from build123d import *

# Parameters (mm, degrees)
SKETCH1_R           = 2.38125
BOSS_EXTRUDE1_DEPTH = 38.1
FILLET1_R           = 2.54
SKETCH2_R           = 6.35
CUT_EXTRUDE1_DEPTH  = 19.05


with BuildPart() as part:
    # Sketch1 → Boss-Extrude1 (new body)
    with BuildSketch(Plane(origin=(0, 0, 0), x_dir=(1, 0, 0), z_dir=(0, 1, 0))):
        with BuildLine():
            Line((216.9989119, 96.687544883), (-5.2510881, 14.137544883))
            ThreePointArc((-5.2510881, 14.137544883), (-14.843448897, -2.667606866), (0, -15.08125))
            Line((0, -15.08125), (241.3, -15.08125))
            ThreePointArc((241.3, -15.08125), (253.102268215, -9.388853313), (255.99503722, 3.391162435))
            Line((255.99503722, 3.391162435), (236.94503722, 85.941162435))
            ThreePointArc((236.94503722, 85.941162435), (229.403197025, 95.826892478), (216.9989119, 96.687544883))
        make_face()
        with Locations(Location((0, 0, 0), (0, 0, 90))):
            Circle(SKETCH1_R, mode=Mode.SUBTRACT)
        with Locations(Location((196.85, 12.7, 0), (0, 0, 90))):
            Circle(SKETCH1_R, mode=Mode.SUBTRACT)
        with Locations(Location((241.3, 0, 0), (0, 0, 90))):
            Circle(SKETCH1_R, mode=Mode.SUBTRACT)
        with Locations(Location((222.25, 82.55, 0), (0, 0, 90))):
            Circle(SKETCH1_R, mode=Mode.SUBTRACT)
    extrude(amount=BOSS_EXTRUDE1_DEPTH)

    # Fillet1
    fillet1_edges = [part.edges().sort_by_distance(p)[0] for p in [
        (229.403197025, 38.1, -95.826892478),
        (253.102268215, 0, 9.388853313),
        (120.65, 0, 15.08125),
        (-14.843448897, 0, 2.667606866),
        (105.8739119, 0, -55.412544883),
        (229.403197025, 0, -95.826892478),
        (246.47003722, 0, -44.666162435),
        (105.8739119, 38.1, -55.412544883),
        (-14.843448897, 38.1, 2.667606866),
        (120.65, 38.1, 15.08125),
        (253.102268215, 38.1, 9.388853313),
        (246.47003722, 38.1, -44.666162435),
    ]]
    fillet(fillet1_edges, radius=FILLET1_R)

    # Sketch2 → Cut-Extrude1 (cut)
    with BuildSketch(Plane(origin=(0, 38.1, 0), x_dir=(1, 0, 0), z_dir=(0, 1, 0))):
        with Locations(Location((0, 0, 0), (0, 0, 270))):
            Circle(SKETCH2_R)
    extrude(amount=-CUT_EXTRUDE1_DEPTH, mode=Mode.SUBTRACT)


solid = part.part
Read the model definition and answer for the solid it produces. Units are mm, in the model's axes. A direction names the side the tool comes from. Round coordinates to 2 decimals unless told otherwise and drop trailing zeros. Loops run counter-clockwise (first coordinate to the right, second up) from the corner with the lowest first, then second, coordinate; pieces in that order, holes last. Notation, with made-up numbers: (-21, 12) - (35, 12) arc R33 ccw to (35, 51) - close; hole circle Ø9 at (10.5, 0). An arc over 180 degrees is marked (long way). One line per question, with ' | ' between items. Start each with the question number.
Q1. Flat-ended cylindrical pins translate along their axes: pin 1 (2 mm diameter, centred on y = 7.5, z = -56.5, fed in from +X); pin 2 (4 mm diameter, centred on x = 60.5, y = 11.5, fed in from -Z); pin 3 (5 mm diameter, centred on y = 33, z = -59.5, fed in from +X); pin 4 (4.5 mm diameter, centred on x = 222.25, z = -82.55, fed in from +Y). Find the tip coordinate at first contact, or state that the pin passes through.
Q2. Find the intervals of material crossed by L1, parallel to X at y = 33.75, z = 0; L2, parallel to X at y = 14, z = -1.5; L3, parallel to X at y = 21, z = -12.7, in increasing order.
Q3. For faces 1 (the flat face through (107.43, 18.82, -55.99)), 2 (the flat face through (0, 19.05, 3)), determine the directions among +Z, -Z, +X, -X, +Y, -Y from which every point of the face is accessible in a straight line to the end or side of a thin tool.
Q4. Section C-C on y = 23.5 is taken. Give the vertices of the cut face in (x, z), plus the area to 3 significant figures.
Q5. Section B-B on z = 0 is taken. Count the separate pieces of the cut face and the enclosed holes in it, plus the area to 3 significant figures.
Q6. For a pull along Z with two mould halves and no side action, classify faces 3 (the cylindrical face through (1.45, 9.39, 1.89)), 4 (the cylindrical face through (-14.893, 18.819, 2.378)), 5 (the flat face through (148, 38.1, -30)) as +Z half, -Z half, draft (parallel to the pull), parting line (faces both ways), or undercut.
Q7. Section A-A on y = 13 is taken. Give the vertices of the cut face in (x, z), plus the area to 3 significant figures.
Established:
1) pin 1: x = 243.97 | pin 2: z = -39.3 | pin 3: x = 243.62 | pin 4: through
2) L1: -15.08 to -6.35, 6.35 to 238.92, 243.68 to 256.38 | L2: -15.01 to -1.85, 1.85 to 239.45, 243.15 to 256.31 | L3: -8.13 to 194.47, 199.23 to 253.85
3) face 1: -Z, -X, +Y, -Y | face 2: +Y
4) outline: (-5.25, -14.14) - (217, -96.69) arc R15.08 ccw to (236.95, -85.94) - (256, -3.39) arc R15.08 ccw to (241.3, 15.08) - (0, 15.08) arc R15.08 ccw to start; hole circle Ø12.7 at (0, 0); hole circle Ø4.76 at (196.85, -12.7); hole circle Ø4.76 at (222.25, -82.55); hole circle Ø4.76 at (241.3, 0) | area: 19,000 mm²
5) separate pieces: 3 | enclosed holes: 0 | area: 9,820 mm²
6) face 3: undercut | face 4: parting line | face 5: draft
7) outline: (-5.25, -14.14) - (217, -96.69) arc R15.08 ccw to (236.95, -85.94) - (256, -3.39) arc R15.08 ccw to (241.3, 15.08) - (0, 15.08) arc R15.08 ccw to start; hole circle Ø4.76 at (0, 0); hole circle Ø4.76 at (196.85, -12.7); hole circle Ø4.76 at (222.25, -82.55); hole circle Ø4.76 at (241.3, 0) | area: 19,100 mm²
